```python
from build123d import *

# Parameters (mm, degrees)
EXTRUDE_1_DEPTH             = 8
HOLE_WIZARD_M41_D           = 4.5
HOLE_WIZARD_M41_CSINK_D     = 9.4
HOLE_WIZARD_M41_CSINK_ANGLE = 90
CUT_EXTRUDE_2_DEPTH         = 5
CHAMFER_1_SIZE              = 3


with BuildPart() as part:
    # Эскиз1 → Бобышка-Вытянуть1 (new, symmetric)
    with BuildSketch(Plane.XY):
        with BuildLine():
            Line((-8, 50.586847211), (8, 50.586847211))
            Line((8, 50.586847211), (8, 34.586847211))
            ThreePointArc((8, 34.586847211), (25.102290732, 25.102290732), (34.586847211, 8))
            Line((34.586847211, 8), (50.586847211, 8))
            Line((50.586847211, 8), (50.586847211, 0.5))
            Line((50.586847211, 0.5), (25.495097568, 0.5))
            ThreePointArc((25.495097568, 0.5), (-25.5, 0), (25.495097568, -0.5))
            Line((25.495097568, -0.5), (50.586847211, -0.5))
            Line((50.586847211, -0.5), (50.586847211, -8))
            Line((50.586847211, -8), (34.586847211, -8))
            ThreePointArc((34.586847211, -8), (25.102290732, -25.102290732), (8, -34.586847211))
            Line((8, -34.586847211), (8, -50.586847211))
            Line((8, -50.586847211), (-8, -50.586847211))
            Line((-8, -50.586847211), (-8, -34.586847211))
            ThreePointArc((-8, -34.586847211), (-25.102290732, -25.102290732), (-34.586847211, -8))
            Line((-34.586847211, -8), (-50.586847211, -8))
            Line((-50.586847211, -8), (-50.586847211, 8))
            Line((-50.586847211, 8), (-34.586847211, 8))
            ThreePointArc((-34.586847211, 8), (-25.102290732, 25.102290732), (-8, 34.586847211))
            Line((-8, 34.586847211), (-8, 50.586847211))
        make_face()
    extrude(amount=EXTRUDE_1_DEPTH, both=True)

    # Зенковка для винта с полупотайной головкой M41 (through all)
    with Locations(Plane(origin=(42.586847211, 8, 0), x_dir=(1, 0, 0), z_dir=(0, 1, 0))):
        with Locations((0, 0)):
            CounterSinkHole(HOLE_WIZARD_M41_D / 2, HOLE_WIZARD_M41_CSINK_D / 2, counter_sink_angle=HOLE_WIZARD_M41_CSINK_ANGLE)

    # Эскиз5 → Вырез-Вытянуть2 (cut)
    with BuildSketch(Plane.XZ.offset(8)):
        Polygon((46.91697423, 0), (44.751910721, 3.75), (40.421783702, 3.75), (38.256720192, 0), (40.421783702, -3.75), (44.751910721, -3.75), align=None)
    extrude(amount=-CUT_EXTRUDE_2_DEPTH, mode=Mode.SUBTRACT)

    # Фаска1
    chamfer_1_edges = [part.edges().sort_by_distance(p)[0] for p in [
        (-25.5, 0, -8),
        (50.586847211, -8, 0),
        (8, -50.586847211, 0),
        (-8, -50.586847211, 0),
        (-50.586847211, -8, 0),
        (-50.586847211, 8, 0),
        (-8, 50.586847211, 0),
        (8, 50.586847211, 0),
        (50.586847211, 8, 0),
        (-25.5, 0, 8),
    ]]
    chamfer(chamfer_1_edges, length=CHAMFER_1_SIZE)


solid = part.part
```
Can you work these out from the model? Positions are in its coordinate system, mm. A direction names the side the tool comes from. Round coordinates to 2 decimals unless told otherwise and drop trailing zeros. Loops run counter-clockwise (first coordinate to the right, second up) from the corner with the lowest first, then second, coordinate; pieces in that order, holes last.
Item 1: Which directions (+Z, -Z, +X, -X, +Y, -Y) give clear straight access to the entire face, cutting with the end or side of a thin tool? Please do faces 1 (the flat face through (0, 50.587, 0)), 2 (the flat face through (8, 41, 0)), 3 (the flat face through (43, -6, 3.75)), 4 (the flat face through (38, 0.5, 0)), 5 (the conical face through (40.327, 5.669, -0.712)).
Item 2: Suppose I cut it at B-B, the plane z = -6.75. Write out the boundary of the cut face in (x, y), then the cut area to 3 significant figures.
Item 3: Will these pins go through, and if not, where does the flat tip stop? pin 1 Ø5 at (x, z) = (42.59, 0) entering from -Y; pin 2 Ø8 at (x, z) = (44.5, 1) entering from -Y; pin 3 Ø4 at (x, z) = (-41, 2) entering from +Y; pin 4 Ø4 at (x, z) = (42.59, 0) entering from +Y.
Item 4: If we mould it in two halves opening along X, with no side actions, what happens to faces 6 (the flat face through (49.066, -6.521, 0.112)), 7 (the flat face through (-49.066, 6.521, 0.112)), 8 (the flat face through (38, -8, 0)), 9 (the cylindrical face through (44.835, -1.768, -0.099))? For each: +X half, -X half, draft (parallel to the pull), parting line (faces both ways), or undercut.
Item 5: Suppose I cut it at A-A, the plane x = 0. Write out the boundary of the cut face in (y, z).
Item 6: Please list where these lines run through material, in increasing order: L1, parallel to Y at x = 0, z = 2.75; L2, parallel to Y at x = 46, z = -4; L3, parallel to X at y = 4.5, z = -0.5.
Reported:
1. face 1: +Z, -Z, +X, -X, +Y
1. face 2: +Z, -Z, +X, +Y
1. face 3: -Y
1. face 4: +Z, -Z, +X
1. face 5: +Y
2. outline: (-50.59, -5) - (-47.59, -8) - (-34.59, -8) arc R35.5 ccw to (-8, -34.59) - (-8, -47.59) - (-5, -50.59) - (5, -50.59) - (8, -47.59) - (8, -34.59) arc R35.5 ccw to (34.59, -8) - (47.59, -8) - (50.59, -5) - (50.59, -0.5) - (27.25, -0.5) arc R27.25 cw (long way) to (27.25, 0.5) - (50.59, 0.5) - (50.59, 5) - (47.59, 8) - (34.59, 8) arc R35.5 ccw to (8, 34.59) - (8, 47.59) - (5, 50.59) - (-5, 50.59) - (-8, 47.59) - (-8, 34.59) arc R35.5 ccw to (-34.59, 8) - (-47.59, 8) - (-50.59, 5) - close
2. area: 2,550 mm2
3. pin 1: stops at y = -3
3. pin 2: stops at y = -8
3. pin 3: stops at y = 8
3. pin 4: passes through
4. face 6: +X half
4. face 7: -X half
4. face 8: draft
4. face 9: undercut
5. outline: (-50.59, -8) - (-28.5, -8) - (-25.5, -5) - (-25.5, 5) - (-28.5, 8) - (-50.59, 8) - close; (25.5, -5) - (28.5, -8) - (50.59, -8) - (50.59, 8) - (28.5, 8) - (25.5, 5) - close
6. L1: y = -50.59 to -25.5, 25.5 to 50.59
6. L2: y = -8 to -0.5, 0.5 to 8
6. L3: x = -50.59 to -25.1, 25.1 to 40.39, 44.78 to 50.59
